For this review, take the finished solid that the model builds, in its own axes (mm). Face numbers are marked on the shaded views. A direction names the side the tool comes from. Coordinates: 2 decimals unless noted, no trailing zeros. Order: outer loops, then holes, each group sorted by start corner. A loop starts at its lowest first (then second) coordinate and runs counter-clockwise, first axis right, second up.
from build123d import *

# Parameters (mm, degrees)
SKETCH_W           = 19.6
SKETCH_H           = 20.312846
SKETCH_R           = 7.6
PAD_DEPTH          = 22
SKETCH002_W        = 17.1
SKETCH002_H        = 8.369387
PAD001_DEPTH       = 8.5
POCKET_DEPTH       = 8
PAD002_DEPTH       = 13.630613
SKETCH005_R        = 1.65
POCKET001_DEPTH    = 8.370387
POCKET002_DEPTH    = 104.4228440614
POLARPATTERN_COUNT = 8
SKETCH010_W        = 2.1
SKETCH010_H        = 22
PAD004_DEPTH       = 1.5
SKETCH011_W        = 1.5
SKETCH011_H        = 8.369387
PAD005_DEPTH       = 0.4
SKETCH012_R        = 1.75
POCKET005_DEPTH    = 4


with BuildPart() as part:
    # Sketch → Pad (new body)
    with BuildSketch(Plane.YZ):
        with Locations((0, 0.656423)):
            Rectangle(SKETCH_W, SKETCH_H)
        Circle(SKETCH_R, mode=Mode.SUBTRACT)
    extrude(amount=-PAD_DEPTH)

    # Sketch002 → Pad001 (join)
    with BuildSketch(Plane(origin=(0, 0, 10.812846), x_dir=(0, -1, 0), z_dir=(0, 0, 1))):
        with Locations((-1.25, -17.8153065)):
            Rectangle(SKETCH002_W, SKETCH002_H)
    extrude(amount=PAD001_DEPTH)

    # Sketch003 → Pocket (cut)
    with BuildSketch(Plane(origin=(0, -7.3, 0), x_dir=(0, 0, -1), z_dir=(0, -1, 0))):
        with BuildLine():
            Line((-12.312846, -22), (-12.312846, -13.630613))
            Line((-12.312846, -13.630613), (-13.4208073614, -13.630613))
            ThreePointArc((-13.912846, -14.0417424305), (-13.5922491229, -13.9254319435), (-13.4208073614, -13.630613))
            ThreePointArc((-13.912846, -14.0417424305), (-14.412846, -14.5417424305), (-13.912846, -15.0417424305))
            ThreePointArc((-13.912846, -16.0417424305), (-13.412846, -15.5417424305), (-13.912846, -15.0417424305))
            ThreePointArc((-13.912846, -16.0417424305), (-14.412846, -16.5417424305), (-13.912846, -17.0417424305))
            ThreePointArc((-13.912846, -18.0417424305), (-13.412846, -17.5417424305), (-13.912846, -17.0417424305))
            ThreePointArc((-13.912846, -18.0417424305), (-14.412846, -18.5417424305), (-13.912846, -19.0417424305))
            ThreePointArc((-13.912846, -20.0417424305), (-13.412846, -19.5417424305), (-13.912846, -19.0417424305))
            ThreePointArc((-13.912846, -20.0417424305), (-14.412846, -20.5417424305), (-13.912846, -21.0417424305))
            ThreePointArc((-13.712846, -22), (-13.4233928435, -21.4395876087), (-13.912846, -21.0417424305))
            Line((-13.712846, -22), (-12.312846, -22))
        make_face()
    extrude(amount=-POCKET_DEPTH, mode=Mode.SUBTRACT)

    # Sketch004 (on Face7 of Pocket) → Pad002 (join)
    with BuildSketch(Plane.YZ.offset(-13.630613)):
        Polygon((9.8, 19.312846), (1.3, 19.312846), (1.3, 18.062846), (8.55, 18.062846), (8.55, 10.812846), (9.8, 10.812846), align=None)
    extrude(amount=PAD002_DEPTH)

    # Sketch005 (on Face7 of Pad002) → Pocket001 (cut, through all)
    with BuildSketch(Plane.YZ.offset(-13.630613)):
        with Locations((4.925, 14.437846)):
            Circle(SKETCH005_R)
    extrude(amount=-POCKET001_DEPTH, mode=Mode.SUBTRACT)

    # Sketch006 (on Face5 of Pocket001) → Pocket002 (cut, through all)
    with BuildSketch(Plane(origin=(-22, 0, 0), x_dir=(0, 1, 0), z_dir=(-1, 0, 0))):
        with BuildLine():
            ThreePointArc((-7.622006143, 3.1571383175), (-8.0914785633, 1.6094951569), (-8.25, 0))
            Line((-7, 0), (-8.25, 0))
            ThreePointArc((-6.4671567274, 2.678784027), (-6.8654969628, 1.3656322543), (-7, 0))
            Line((-6.4671567274, 2.678784027), (-7.622006143, 3.1571383175))
        make_face()
    pocket002 = extrude(amount=-POCKET002_DEPTH, mode=Mode.SUBTRACT)

    # PolarPattern: Pocket002 ×8 about axis
    polarpattern_axis = Axis((0, 0, 0), (1, 0, 0))
    for i in range(1, POLARPATTERN_COUNT):
        add(pocket002.rotate(polarpattern_axis, i * 360 / POLARPATTERN_COUNT), mode=Mode.SUBTRACT)

    # Sketch010 (on Face2 of PolarPattern) → Pad004 (join)
    with BuildSketch(Plane(origin=(0, 0, 10.812846), x_dir=(0, -1, 0), z_dir=(0, 0, 1))):
        with Locations((8.75, -11)):
            Rectangle(SKETCH010_W, SKETCH010_H)
    extrude(amount=PAD004_DEPTH)

    # Sketch011 (on Face52 of Pad004) → Pad005 (join)
    with BuildSketch(Plane(origin=(0, -7.3, 0), x_dir=(0, 0, -1), z_dir=(0, -1, 0))):
        with Locations((-11.562846, -17.8153065)):
            Rectangle(SKETCH011_W, SKETCH011_H)
    extrude(amount=PAD005_DEPTH)

    # Sketch012 (on Face2 of Pad005) → Pocket005 (cut)
    with BuildSketch(Plane.ZX.offset(9.8)):
        with Locations((8.062846, -3.5)):
            Circle(SKETCH012_R)
        with Locations((8.062846, -18.5)):
            Circle(SKETCH012_R)
    extrude(amount=-POCKET005_DEPTH, mode=Mode.SUBTRACT)


solid = part.part
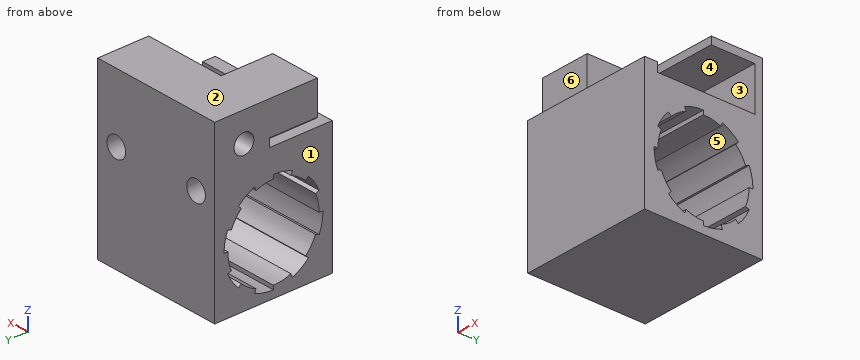
1. Take a section at D-D, the plane x = -18.5. Give the number of separate pieces and of enclosed holes in the cut face, plus the area to 3 significant figures.
Answer below:
separate pieces: 1
enclosed holes: 2
area: 310 mm2
2. To check wall thickness, follow L1, parallel to Z at x = -0.75, y = 8.5; L2, parallel to Z at x = -9.75, y = 4.25; L3, parallel to Z at x = -13.5, y = 5.75. State the ranges of each line that lie inside material, in increasing order.
Answer below:
L1: z = -9.5 to 10.81, 18.06 to 19.31
L2: z = -9.5 to -6.3, 7.07 to 10.81, 18.06 to 19.31
L3: z = -9.5 to -5.75, 4.97 to 5.75, 5.92 to 10.81, 18.06 to 19.31
3. Take a section at B-B, the plane z = -1.5. Give the boundary of the cut face in (x, y).
Answer below:
outline: (-22, -9.8) - (0, -9.8) - (0, -8.11) - (-22, -8.11) - close; (-22, 7.45) - (0, 7.45) - (0, 9.8) - (-22, 9.8) - close
4. Machinability: for the marked faces 4, 5 and 6, which of the approach directions +Z, -Z, +X, -X, +Y, -Y give a long, thin tool a straight path to every point of the face, cutting with its end or side? Answer none if there is none.
Answer below:
face 4: +X, -Y
face 5: +X, -X
face 6: +Z, +X, -X, -Y
5. Clearance check with flat-ended pins moving along their axes: pin 1 Ø4.5 at (y, z) = (4.92, 14.44) entering from +X; pin 2 Ø4.5 at (x, z) = (-16, 16) entering from -Y; pin 3 Ø4 at (y, z) = (7, -6) entering from +X; pin 4 Ø1.5 at (x, y) = (-2.5, -2) entering from +Z. State where each tip first meets the part, or that it passes through.
Answer below:
pin 1: stops at x = -13.63
pin 2: stops at y = -7.3
pin 3: stops at x = 0
pin 4: stops at z = 10.81
6. The part is to be moulded in two halves that separate along Z. For the marked faces 1, 2 and 3, say which applies: +Z half, -Z half, draft (parallel to the pull), parting line (faces both ways), or undercut.
Answer below:
face 1: draft
face 2: +Z half
face 3: undercut
7. Take a section at C-C, the plane y = -0.5. Give the boundary of the cut face in (x, z).
Answer below:
outline: (-22, -9.5) - (0, -9.5) - (0, -7.58) - (-22, -7.58) - close; (-22, 8.23) - (0, 8.23) - (0, 10.81) - (-13.63, 10.81) - (-13.63, 12.31) - (-22, 12.31) - close; (-22, 13.71) arc R0.5 ccw to (-21.04, 13.91) arc R0.5 cw to (-20.04, 13.91) arc R0.5 ccw to (-19.04, 13.91) arc R0.5 cw to (-18.04, 13.91) arc R0.5 ccw to (-17.04, 13.91) arc R0.5 cw to (-16.04, 13.91) arc R0.5 ccw to (-15.04, 13.91) arc R0.5 cw to (-14.04, 13.91) arc R0.5 ccw to (-13.63, 13.42) - (-13.63, 19.31) - (-22, 19.31) - close
8. Take a section at A-A, the plane y = -4.5. Give the boundary of the cut face in (x, z), plus the area to 3 significant figures.
Answer below:
outline: (-22, -9.5) - (0, -9.5) - (0, -6.91) - (-22, -6.91) - close; (-22, 6.12) - (0, 6.12) - (0, 10.81) - (-13.63, 10.81) - (-13.63, 12.31) - (-22, 12.31) - close; (-22, 13.71) arc R0.5 ccw to (-21.04, 13.91) arc R0.5 cw to (-20.04, 13.91) arc R0.5 ccw to (-19.04, 13.91) arc R0.5 cw to (-18.04, 13.91) arc R0.5 ccw to (-17.04, 13.91) arc R0.5 cw to (-16.04, 13.91) arc R0.5 ccw to (-15.04, 13.91) arc R0.5 cw to (-14.04, 13.91) arc R0.5 ccw to (-13.63, 13.42) - (-13.63, 19.31) - (-22, 19.31) - close
area: 218 mm2
